Read the model definition and answer for the solid it produces. Units are mm, in the model's axes. Give positions to 0.01 mm unless a question says otherwise; leave off trailing zeros. Order: outer loops, then holes, each group sorted by start corner. A loop starts at its lowest first (then second) coordinate and runs counter-clockwise, first axis right, second up. Notation, with made-up numbers: (41, 58.5) - (48, 58.5) arc R8 cw to (48, 63.5) - close; hole circle Ø7 at (68, 74.25). An arc over 180 degrees is marked (long way). Return JSON: item names as keys, results as strings.
```python
from build123d import *

# Parameters (mm, degrees)
SKETCH1_W           = 150
SKETCH1_H           = 200
BOSS_EXTRUDE1_DEPTH = 3
BUTTONS_R           = 6
BUTTONS_R_2         = 6.5
BUTTONS_R_3         = 3.5
CUT_EXTRUDE2_DEPTH  = 126.035994817
CUT_EXTRUDE3_DEPTH  = 1
BOXHOLES_R          = 1.5
BOX_HOLES_CUT_DEPTH = 126.035994817


with BuildPart() as part:
    # Sketch1 → Boss-Extrude1 (new body)
    with BuildSketch(Plane(origin=(0, 0, 0), x_dir=(1, 0, 0), z_dir=(0, 1, 0))):
        Rectangle(SKETCH1_W, SKETCH1_H)
    extrude(amount=BOSS_EXTRUDE1_DEPTH)

    # Buttons → Cut-Extrude2 (cut, through all)
    with BuildSketch(Plane(origin=(0, 3, 0), x_dir=(1, 0, 0), z_dir=(0, 1, 0))):
        with Locations(Location((-55, 70, 0), (0, 0, 270))):
            Circle(BUTTONS_R)
        with Locations(Location((-25, 70, 0), (0, 0, 270))):
            Circle(BUTTONS_R)
        with Locations(Location((0, 70, 0), (0, 0, 270))):
            Circle(BUTTONS_R)
        with Locations(Location((55, 70, 0), (0, 0, 270))):
            Circle(BUTTONS_R)
        with Locations(Location((55, 35, 0), (0, 0, 270))):
            Circle(BUTTONS_R_2)
        with Locations(Location((25, 35, 0), (0, 0, 270))):
            Circle(BUTTONS_R_2)
        with Locations(Location((55, -55, 0), (0, 0, 270))):
            Circle(BUTTONS_R_2)
        with Locations(Location((-55, 40, 0), (0, 0, 270))):
            Circle(BUTTONS_R_3)
        with Locations(Location((-5, 40, 0), (0, 0, 270))):
            Circle(BUTTONS_R_3)
        with Locations(Location((-30, 40, 0), (0, 0, 270))):
            Circle(BUTTONS_R_3)
        with Locations(Location((55, -85, 0), (0, 0, 270))):
            Circle(BUTTONS_R_2)
        with Locations(Location((20, -85, 0), (0, 0, 270))):
            Circle(BUTTONS_R_2)
        with Locations(Location((20, -55, 0), (0, 0, 270))):
            Circle(BUTTONS_R_3)
        with Locations(Location((-60, -55, 0), (0, 0, 270))):
            Circle(BUTTONS_R_3)
        with Locations(Location((-30, -55, 0), (0, 0, 270))):
            Circle(BUTTONS_R_3)
        with Locations(Location((-60, -85, 0), (0, 0, 270))):
            Circle(BUTTONS_R_3)
        with Locations(Location((-30, -85, 0), (0, 0, 270))):
            Circle(BUTTONS_R_3)
        with Locations(Location((-45, -70, 0), (0, 0, 270))):
            Circle(BUTTONS_R_2)
        with Locations(Location((30, 0, 0), (0, 0, 270))):
            Circle(BUTTONS_R_2)
        with Locations(Location((55, 0, 0), (0, 0, 270))):
            Circle(BUTTONS_R_2)
        with Locations(Location((35, -25, 0), (0, 0, 270))):
            Circle(BUTTONS_R_3)
        with Locations(Location((55, -25, 0), (0, 0, 270))):
            Circle(BUTTONS_R_3)
        with Locations(Location((15, -25, 0), (0, 0, 270))):
            Circle(BUTTONS_R_3)
        with Locations(Location((-60, 4, 0), (0, 0, 270))):
            Circle(BUTTONS_R_2)
        with Locations(Location((-37, 4, 0), (0, 0, 270))):
            Circle(BUTTONS_R_2)
        with Locations(Location((-14, 4, 0), (0, 0, 270))):
            Circle(BUTTONS_R_2)
        with Locations(Location((-60, -24, 0), (0, 0, 270))):
            Circle(BUTTONS_R_2)
        with Locations(Location((-37, -24, 0), (0, 0, 270))):
            Circle(BUTTONS_R_2)
        with Locations(Location((-14, -24, 0), (0, 0, 270))):
            Circle(BUTTONS_R_2)
        with Locations(Location((25, 70, 0), (0, 0, 270))):
            Circle(BUTTONS_R)
        with Locations(Location((-15, -70, 0), (0, 0, 270))):
            Circle(BUTTONS_R_2)
    extrude(amount=-CUT_EXTRUDE2_DEPTH, mode=Mode.SUBTRACT)

    # Sketch3 → Cut-Extrude3 (cut)
    with BuildSketch(Plane(origin=(0, 3, 0), x_dir=(1, 0, 0), z_dir=(0, 1, 0))):
        Polygon((75, -40), (1, -40), (1, -100), (-1, -100), (-1, -40), (-75, -40), (-75, -38), (-1, -38), (-1, 17), (-75, 17), (-75, 19), (75, 19), (75, 17), (1, 17), (1, -38), (75, -38), align=None)
    extrude(amount=-CUT_EXTRUDE3_DEPTH, mode=Mode.SUBTRACT)

    # BoxHoles → Box Holes Cut (cut, through all)
    with BuildSketch(Plane(origin=(0, 3, 0), x_dir=(1, 0, 0), z_dir=(0, 1, 0))):
        with Locations(Location((-70, 95, 0), (0, 0, 270))):
            Circle(BOXHOLES_R)
        with Locations(Location((70, 95, 0), (0, 0, 270))):
            Circle(BOXHOLES_R)
        with Locations(Location((70, 0, 0), (0, 0, 270))):
            Circle(BOXHOLES_R)
        with Locations(Location((-70, 0, 0), (0, 0, 270))):
            Circle(BOXHOLES_R)
        with Locations(Location((-70, -95, 0), (0, 0, 270))):
            Circle(BOXHOLES_R)
        with Locations(Location((70, -95, 0), (0, 0, 270))):
            Circle(BOXHOLES_R)
        with Locations(Location((0, 95, 0), (0, 0, 270))):
            Circle(BOXHOLES_R)
        with Locations(Location((0, -95, 0), (0, 0, 270))):
            Circle(BOXHOLES_R)
    extrude(amount=-BOX_HOLES_CUT_DEPTH, mode=Mode.SUBTRACT)


solid = part.part
```
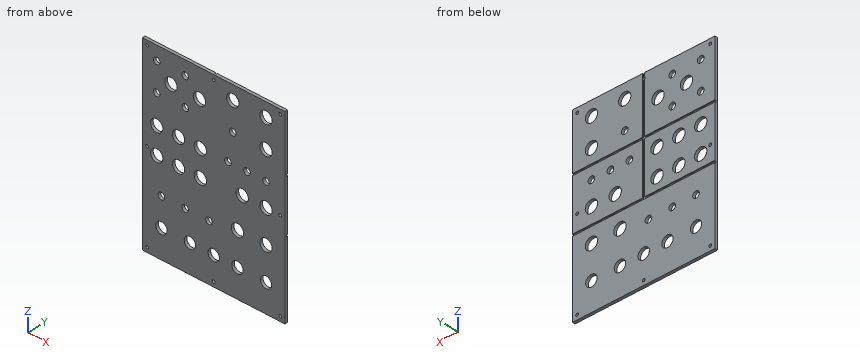
Q1. Consider L1, parallel to X at y = 2.3, z = -70; L2, parallel to X at y = 2.75, z = 85; L3, parallel to X at y = 1.45, z = -9.5. Determine where each line is inside the solid, lowest interval first.
Values:
{"L1": "x = -75 to -61, -49 to -31, -19 to -6, 6 to 19, 31 to 49, 61 to 75", "L2": "x = -75 to -63.5, -56.5 to -33.5, -26.5 to -1, 1 to 13.5, 26.5 to 48.5, 61.5 to 75", "L3": "x = -75 to -63.46, -56.54 to -40.46, -33.54 to -17.46, -10.54 to 75"}
Q2. A cutting plane is placed at B-B (z = 25). Give the number of separate pieces and of enclosed holes in the cut face, and give its area (3 significant figures).
Values:
{"separate pieces": "7", "enclosed holes": "0", "area": "269 mm²"}
Q3. A cutting plane is placed at A-A (z = -70). Write down the section's boundary in (x, y), and give its area (3 significant figures).
Values:
{"outline": "(-75, 0) - (-61, 0) - (-61, 3) - (-75, 3) - close; (-49, 0) - (-31, 0) - (-31, 3) - (-49, 3) - close; (-19, 0) - (-6, 0) - (-6, 3) - (-19, 3) - close; (6, 0) - (19, 0) - (19, 3) - (6, 3) - close; (31, 0) - (49, 0) - (49, 3) - (31, 3) - close; (61, 0) - (75, 0) - (75, 3) - (61, 3) - close", "area": "270 mm²"}
